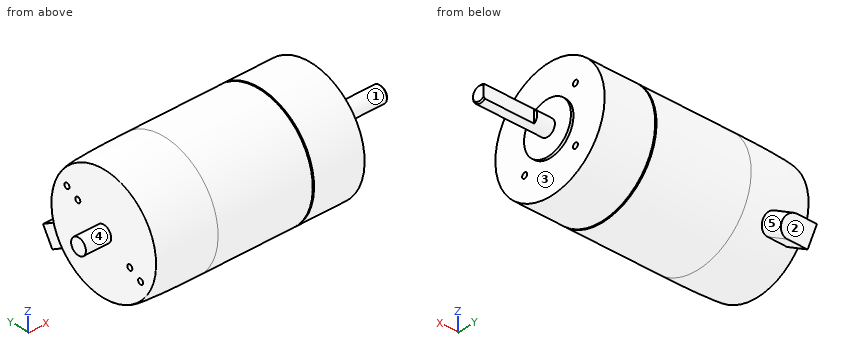
from build123d import *

# Parameters (mm, degrees)
FILLET1_SIZE                   = 1.27
FILLET1_SIZE_2                 = 29.972
SKETCH3_W                      = 6.381173482
SKETCH3_H                      = 3.175
CUT_EXTRUDE1_DEPTH             = 25.4
F_6_32_TAPPED_HOLE2_AT_2_COUNT = 2
F_6_32_TAPPED_HOLE2_AT_2_PITCH = 27.497544243
F_6_32_TAPPED_HOLE2_AT_3_COUNT = 2
F_6_32_TAPPED_HOLE2_AT_3_PITCH = 38.8874
F_6_32_TAPPED_HOLE2_AT_4_COUNT = 2
F_6_32_TAPPED_HOLE2_AT_4_PITCH = 27.497544243
F_6_32_TAPPED_HOLE1_AT_2_COUNT = 2
F_6_32_TAPPED_HOLE1_AT_2_PITCH = 46.0248
F_6_32_TAPPED_HOLE1_AT_3_COUNT = 2
F_6_32_TAPPED_HOLE1_AT_3_PITCH = 39.2684
F_6_32_TAPPED_HOLE1_AT_4_COUNT = 2
F_6_32_TAPPED_HOLE1_AT_4_PITCH = 6.7564
BOSS_EXTRUDE1_DEPTH            = 41.402


with BuildPart() as part:
    # Sketch2 → Revolve1 (revolve)
    with BuildSketch(Plane.XY, mode=Mode.PRIVATE) as revolve1_sk:
        Polygon((35.56, 0), (-116.2558, 0), (-116.2558, 4), (-103.5558, 4), (-103.5558, 29.591), (-26.035, 29.591), (-25.4, 28.956), (-25.4, 29.591), (0, 29.591), (0, 12.7), (1.27, 12.7), (1.27, 4), (34.925, 4), (35.56, 3.365), align=None)
    revolve(revolve1_sk.sketch.rotate(Axis((88.99, 0, 0), (-1, 0, 0)), 90), axis=Axis((88.99, 0, 0), (-1, 0, 0)))

    # Fillet1
    # an asymmetric fillet: 29.972, 1.27 mm, written as the material it takes off along each edge
    with BuildSketch(Plane(origin=(-103.5558, 0, 0), x_dir=(0, 0, -1), z_dir=(0, 1, 0))) as fillet1_piece_1:
        with BuildLine():
            Bezier((29.591 - FILLET1_SIZE, 0), (29.591, 0), (29.591, -FILLET1_SIZE_2), weights=[1, 0.707106781, 1])
            Line((29.591, -FILLET1_SIZE_2), (29.591, 0))
            Line((29.591, 0), (29.591 - FILLET1_SIZE, 0))
        make_face()
    revolve(axis=Axis((-103.5558, 0, 0), (-1, 0, 0)), mode=Mode.SUBTRACT)

    # Sketch3 → Cut-Extrude1 (cut)
    with BuildSketch(Plane(origin=(35.56, 0, 0), x_dir=(0, 0, -1), z_dir=(1, 0, 0))):
        with Locations((0, 4)):
            Rectangle(SKETCH3_W, SKETCH3_H)
    extrude(amount=-CUT_EXTRUDE1_DEPTH, mode=Mode.SUBTRACT)

    # Sketch8 → #6-32 Tapped Hole2 (revolve, cut)
    with BuildSketch(Plane(origin=(0, 13.748772121, 13.748772121), x_dir=(0, 0, -1), z_dir=(0, 1, 0))):
        Polygon((0, 0), (0, 8.81270343), (1.35255, 8.0000094), (1.35255, 0), align=None)
    f_6_32_tapped_hole2 = revolve(axis=Axis((6.35, 13.748772121, 13.748772121), (-1, 0, 0)), mode=Mode.SUBTRACT)

    # #6-32 Tapped Hole2 at 2: #6-32 Tapped Hole2 ×2
    with Locations(*[(0, 0, -i * F_6_32_TAPPED_HOLE2_AT_2_PITCH) for i in range(1, F_6_32_TAPPED_HOLE2_AT_2_COUNT)]):
        add(f_6_32_tapped_hole2, mode=Mode.SUBTRACT)

    # #6-32 Tapped Hole2 at 3: #6-32 Tapped Hole2 ×2
    with Locations(*[Vector(0, -0.7071067811865461, -0.7071067811865489) * (i * F_6_32_TAPPED_HOLE2_AT_3_PITCH) for i in range(1, F_6_32_TAPPED_HOLE2_AT_3_COUNT)]):
        add(f_6_32_tapped_hole2, mode=Mode.SUBTRACT)

    # #6-32 Tapped Hole2 at 4: #6-32 Tapped Hole2 ×2
    with Locations(*[(0, -i * F_6_32_TAPPED_HOLE2_AT_4_PITCH, 0) for i in range(1, F_6_32_TAPPED_HOLE2_AT_4_COUNT)]):
        add(f_6_32_tapped_hole2, mode=Mode.SUBTRACT)

    # Sketch7 → #6-32 Tapped Hole1 (revolve, cut)
    with BuildSketch(Plane(origin=(-103.5558, -19.929323002, -11.5062), x_dir=(0, 0, 1), z_dir=(0, 1, 0))):
        Polygon((0, 0), (0, 10.21069403), (1.35255, 9.398), (1.35255, 0), align=None)
    f_6_32_tapped_hole1 = revolve(axis=Axis((-109.9058, -19.929323002, -11.5062), (1, 0, 0)), mode=Mode.SUBTRACT)

    # #6-32 Tapped Hole1 at 2: #6-32 Tapped Hole1 ×2
    with Locations(*[Vector(0, 0.8660254037844364, 0.5000000000000039) * (i * F_6_32_TAPPED_HOLE1_AT_2_PITCH) for i in range(1, F_6_32_TAPPED_HOLE1_AT_2_COUNT)]):
        add(f_6_32_tapped_hole1, mode=Mode.SUBTRACT)

    # #6-32 Tapped Hole1 at 3: #6-32 Tapped Hole1 ×2
    with Locations(*[Vector(0, 0.8660254037844366, 0.5000000000000038) * (i * F_6_32_TAPPED_HOLE1_AT_3_PITCH) for i in range(1, F_6_32_TAPPED_HOLE1_AT_3_COUNT)]):
        add(f_6_32_tapped_hole1, mode=Mode.SUBTRACT)

    # #6-32 Tapped Hole1 at 4: #6-32 Tapped Hole1 ×2
    with Locations(*[Vector(0, 0.8660254037844365, 0.5000000000000039) * (i * F_6_32_TAPPED_HOLE1_AT_4_PITCH) for i in range(1, F_6_32_TAPPED_HOLE1_AT_4_COUNT)]):
        add(f_6_32_tapped_hole1, mode=Mode.SUBTRACT)

    # Sketch12 → Boss-Extrude1 (add)
    with BuildSketch(Plane(origin=(0, 0, 0), x_dir=(1, 0, 0), z_dir=(0, 0.866025403784438, -0.500000000000001))):
        with BuildLine():
            Line((-98.4758, -5.08), (-88.3158, -5.08))
            ThreePointArc((-88.3158, -5.08), (-83.2358, 0), (-88.3158, 5.08))
            Line((-88.3158, 5.08), (-98.4758, 5.08))
            Line((-98.4758, 5.08), (-98.4758, -5.08))
        make_face()
    extrude(amount=BOSS_EXTRUDE1_DEPTH)


solid = part.part
CAD build for the part. Positions are in the model's coordinates, mm. Face numbers are marked on the shaded views. A direction names the side the tool comes from. Round coordinates to 2 decimals unless told otherwise and drop trailing zeros. Loops run counter-clockwise (first coordinate to the right, second up) from the corner with the lowest first, then second, coordinate; pieces in that order, holes last.
(1) Wall check: line 1 along X through (y, z) = (18, -16); line 2 along X through (y, z) = (-2, 6.5); line 3 along Z through (x, y) = (-37, 14). Give the ranges that are in metal, low to high.
(2) Two-plate mould, pull along Y, no slides. Class the marked faces 3, 4 and 5: +Y half, -Y half, draft (parallel to the pull), parting line (faces both ways), or undercut.
(3) Drop flat-ended pins along their axis: pin 1 (6 mm diameter, centred on y = 3, z = -16, fed in from -X); pin 2 (4 mm diameter, centred on x = -33.5, z = -11, fed in from -Y); pin 3 (3 mm diameter, centred on x = 25.5, z = 0, fed in from +Y). Give the stop position or say it passes through.
(4) Cut at B-B (x = 14.5). Give the cut face in (y, z), plus the area to 3 significant figures.
(5) Which spindle directions (+Z, -Z, +X, -X, +Y, -Y) get a long thin tool onto all of the face, cutting with end or side? Do the marked faces 1 and 2. Say none if no direction does.
(6) Cut at A-A (x = -68.5). Give the cut face in (y, z).
Findings below:
1. line 1: x = -103.56 to 0
1. line 2: x = -103.56 to 1.27
1. line 3: z = -26.07 to 26.07
2. face 3: draft
2. face 4: parting line
2. face 5: undercut
3. pin 1: stops at x = -103.56
3. pin 2: stops at y = -28.19
3. pin 3: stops at y = 2.41
4. outline: (2.41, -3.19) - (2.41, 3.19) arc R4 ccw (long way) to start
4. area: 43.2 mm2
5. face 1: +X
5. face 2: -Z, +X, -X, +Y
6. outline: circle Ø59.18 at (0, 0)
